from build123d import *

# Parameters (mm, degrees)
F0_W     = 2.1
F0_H     = 2.1
F1_DEPTH = 30
F4_DEPTH = 34
F5_DEPTH = 27.5
F6_DEPTH = 7.5


with BuildPart() as f1:
    # F0 (on Top) → F1 (new body)
    with BuildSketch(Plane.XY):
        with BuildLine():
            Line((86, -35), (90, -35))
            Line((90, -35), (90, -23))
            Line((90, -23), (90, 23))
            Line((90, 23), (90, 35))
            Line((90, 35), (86, 35))
            Line((86, 35), (80, 35))
            Line((80, 35), (70.1, 35))
            Line((70.1, 35), (70.1, 22.207107))
            Line((70.1, 22.207107), (72.989087, 25.096194))
            ThreePointArc((72.989087, 25.096194), (73.475722, 25.421353), (74.049747, 25.535534))
            Line((74.049747, 25.535534), (74.635534, 25.535534))
            ThreePointArc((74.635534, 25.535534), (75.696194, 25.096194), (76.135534, 24.035534))
            Line((76.135534, 24.035534), (76.135534, 10.964466))
            ThreePointArc((76.135534, 10.964466), (75.696194, 9.903806), (74.635534, 9.464466))
            Line((74.635534, 9.464466), (74.049747, 9.464466))
            ThreePointArc((74.049747, 9.464466), (73.475722, 9.578647), (72.989087, 9.903806))
            Line((72.989087, 9.903806), (70.1, 12.792893))
            Line((70.1, 12.792893), (70.1, -12.792893))
            Line((70.1, -12.792893), (72.989087, -9.903806))
            ThreePointArc((72.989087, -9.903806), (73.475722, -9.578647), (74.049747, -9.464466))
            Line((74.049747, -9.464466), (74.635534, -9.464466))
            ThreePointArc((74.635534, -9.464466), (75.696194, -9.903806), (76.135534, -10.964466))
            Line((76.135534, -10.964466), (76.135534, -24.035534))
            ThreePointArc((76.135534, -24.035534), (75.696194, -25.096194), (74.635534, -25.535534))
            Line((74.635534, -25.535534), (74.049747, -25.535534))
            ThreePointArc((74.049747, -25.535534), (73.475722, -25.421353), (72.989087, -25.096194))
            Line((72.989087, -25.096194), (70.1, -22.207107))
            Line((70.1, -22.207107), (70.1, -35))
            Line((70.1, -35), (80, -35))
            Line((80, -35), (86, -35))
        make_face()
        Polygon((86, 35), (90, 35), (90, 37.1), (70.1, 37.1), (70.1, 35), (80, 35), align=None)
        Polygon((90, -23), (90, -35), (92.1, -35), (92.1, 35), (90, 35), (90, 23), align=None)
        with Locations((91.05, 36.05)):
            Rectangle(F0_W, F0_H)
        Polygon((92.1, 35), (92.1, -35), (92.1, -37.1), (125.1, -37.1), (125.1, 37.1), (92.1, 37.1), align=None)
        Polygon((90, -37.1), (90, -35), (86, -35), (80, -35), (70.1, -35), (70.1, -37.1), align=None)
        with Locations((91.05, -36.05)):
            Rectangle(F0_W, F0_H)
    extrude(amount=F1_DEPTH)

    # F3 (on Front) → F4 (cut, symmetric)
    with BuildSketch(Plane.XZ):
        Polygon((105, 26), (79, 0), (125.1, 0), (125.1, 26), align=None)
    extrude(amount=F4_DEPTH, both=True, mode=Mode.SUBTRACT)

    # F3 (on Front) → F5 (cut, symmetric)
    with BuildSketch(Plane.XZ):
        Polygon((105, 26), (79, 0), (125.1, 0), (125.1, 26), align=None)
        Polygon((85, 26), (79, 0), (105, 26), align=None)
    extrude(amount=F5_DEPTH, both=True, mode=Mode.SUBTRACT)

    # F3 (on Front) → F6 (join, symmetric)
    with BuildSketch(Plane.XZ):
        Polygon((85, 26), (79, 0), (105, 26), align=None)
    extrude(amount=F6_DEPTH, both=True)


solid = f1.part
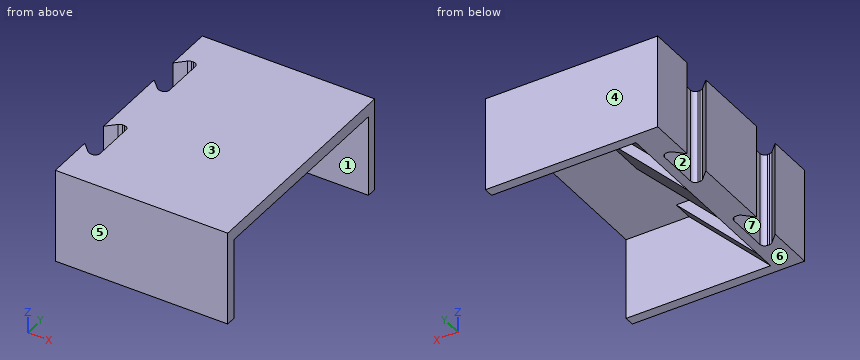
Check sheet for the modelled part. Datum: model origin and axes. Units: mm. Face numbers are marked on the shaded views. A direction names the side the tool comes from. Round coordinates to 2 decimals unless told otherwise and drop trailing zeros. Loops run counter-clockwise (first coordinate to the right, second up) from the corner with the lowest first, then second, coordinate; pieces in that order, holes last.
1. Sectioned sample at B-B on z = 28. Record the boundary of the cut face in (x, y).
2. Sectioned sample at D-D on x = 89.5. Record the boundary of the cut face in (y, z).
3. Sectioned sample at A-A on x = 98. Record the boundary of the cut face in (y, z), and give its area (3 significant figures).
4. Sectioned sample at C-C on y = 15.5. Record the boundary of the cut face in (x, z).
5. Gauge pin test, flat ends, axial feed: pin 1 Ø4 at (y, z) = (-19.5, 5.5) entering from +X; pin 2 Ø10 at (x, y) = (96.5, -8.5) entering from -Z; pin 3 Ø12 at (y, z) = (-1.5, 13.5) entering from +X. Record the tip position at first contact, or that the pin passes through.
6. Set-up check for the marked faces 1, 2 and 3: record each of +Z, -Z, +X, -X, +Y, -Y from which the full face is reachable in a straight line by a thin tool's end or side.
7. Mould release check, pull along Y, two halves, no side actions. Record for the marked faces 4, 5, 6 and 7: released by +Y, released by -Y, zero draft, split by the parting line, or undercut.
8. Scan lines: probe 1 along Y at (x, z) = (114.5, 22); probe 2 along Y at (x, z) = (82, 4.5); probe 3 along Y at (x, z) = (74, 4). Record each from-to range of solid material in increasing order.
Recorded:
1. outline: (70.1, -37.1) - (125.1, -37.1) - (125.1, 37.1) - (70.1, 37.1) - (70.1, 22.21) - (72.99, 25.1) arc R1.5 cw to (74.05, 25.54) - (74.64, 25.54) arc R1.5 cw to (76.14, 24.04) - (76.14, 10.96) arc R1.5 cw to (74.64, 9.46) - (74.05, 9.46) arc R1.5 cw to (72.99, 9.9) - (70.1, 12.79) - (70.1, -12.79) - (72.99, -9.9) arc R1.5 cw to (74.05, -9.46) - (74.64, -9.46) arc R1.5 cw to (76.14, -10.96) - (76.14, -24.04) arc R1.5 cw to (74.64, -25.54) - (74.05, -25.54) arc R1.5 cw to (72.99, -25.1) - (70.1, -22.21) - close
2. outline: (-37.1, 0) - (-34, 0) - (-34, 10.5) - (-27.5, 10.5) - (-27.5, 26) - (-7.5, 26) - (-7.5, 10.5) - (7.5, 10.5) - (7.5, 26) - (27.5, 26) - (27.5, 10.5) - (34, 10.5) - (34, 0) - (37.1, 0) - (37.1, 30) - (-37.1, 30) - close
3. outline: (-37.1, 0) - (-34, 0) - (-34, 19) - (-27.5, 19) - (-27.5, 26) - (-7.5, 26) - (-7.5, 19) - (7.5, 19) - (7.5, 26) - (27.5, 26) - (27.5, 19) - (34, 19) - (34, 0) - (37.1, 0) - (37.1, 30) - (-37.1, 30) - close
3. area: 654 mm2
4. outline: (76.14, 0) - (79, 0) - (85, 26) - (125.1, 26) - (125.1, 30) - (76.14, 30) - close
5. pin 1: stops at x = 80.73
5. pin 2: stops at z = 12.6
5. pin 3: stops at x = 98.5
6. face 1: -Z, +X
6. face 2: +Z, -Z
6. face 3: +Z, +X, -X, +Y, -Y
7. face 4: released by +Y
7. face 5: released by -Y
7. face 6: zero draft
7. face 7: undercut
8. probe 1: y = -37.1 to -34, 34 to 37.1
8. probe 2: y = -37.1 to -27.5, -7.5 to 7.5, 27.5 to 37.1
8. probe 3: y = -37.1 to -25.53, -9.47 to 9.47, 25.53 to 37.1
